Here's how the part is built. I have some questions about the finished solid (model axes, mm). Face numbers are marked on the shaded views. A direction names the side the tool comes from. Give positions to 0.01 mm unless a question says otherwise; leave off trailing zeros. Order: outer loops, then holes, each group sorted by start corner. A loop starts at its lowest first (then second) coordinate and runs counter-clockwise, first axis right, second up. Notation, with made-up numbers: (-4, 40) - (9, 40) arc R25 ccw to (9, 70) - close; hole circle Ø10 at (34.25, -3). An arc over 180 degrees is marked (long way). One line per question, with ' | ' between items.
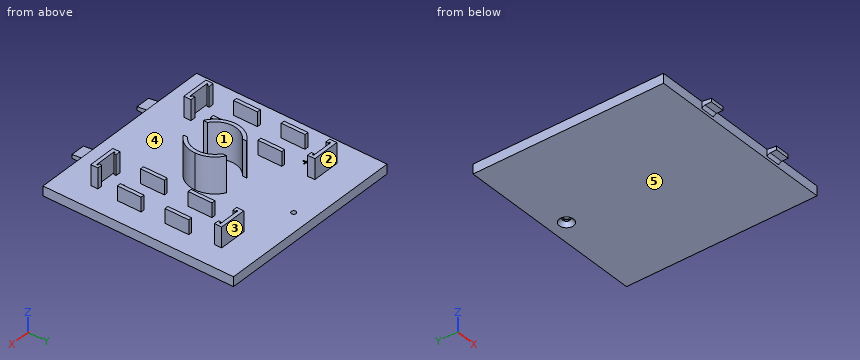
from build123d import *

# Parameters (mm, degrees)
F1_DEPTH       = 4
F2_W           = 1.5
F2_H           = 10
F3_DEPTH       = 6
F2_W_2         = 7.5
F2_H_2         = 1.5
F4_DEPTH       = 8.5
F5_R           = 1
F6_DEPTH       = 25
F7_START       = -2
F5_R_2         = 1.5
F7_DEPTH       = 23
F8_SIZE        = 1.5
F10_DEPTH      = 40
F10_DEPTH_BACK = 40
F0_W           = 20
F0_H           = 4
F0_W_2         = 28
F11_DEPTH      = 18.6
F12_DEPTH      = 0.3
F14_DEPTH      = 15


with BuildPart() as f1:
    # F0 (on Top) → F1 (new body)
    with BuildSketch(Plane.XY):
        Polygon((40, 40), (-40, 40), (-40, -40), (-20, -40), (-14, -40), (14, -40), (20, -40), (40, -40), align=None)
    extrude(amount=F1_DEPTH)

    # F2 (on face) → F3 (join)
    with BuildSketch(Plane.XY.offset(4)):
        with Locations((-30.3, -11)):
            Rectangle(F2_W, F2_H)
        with Locations((-18.2, -11)):
            Rectangle(F2_W, F2_H)
        with Locations((-18.2, 9)):
            Rectangle(F2_W, F2_H)
        with Locations((-30.3, 9)):
            Rectangle(F2_W, F2_H)
        with Locations((18.2, -11)):
            Rectangle(F2_W, F2_H)
        with Locations((18.2, 9)):
            Rectangle(F2_W, F2_H)
        with Locations((30.3, 9)):
            Rectangle(F2_W, F2_H)
        with Locations((30.3, -11)):
            Rectangle(F2_W, F2_H)
    extrude(amount=F3_DEPTH)

    # F2 (on face) → F4 (join)
    with BuildSketch(Plane.XY.offset(4)):
        Polygon((-28, 27), (-30, 27), (-30, 24), (-28, 24), (-28, 25), (-28.75, 25), (-28.75, 25.5), (-28, 25.5), align=None)
        with Locations((-24.25, 26.25)):
            Rectangle(F2_W_2, F2_H_2)
        Polygon((-18.5, 27), (-20.5, 27), (-20.5, 25.5), (-19.75, 25.5), (-19.75, 25), (-20.5, 25), (-20.5, 24), (-18.5, 24), align=None)
        Polygon((-20.5, -28), (-18.5, -28), (-18.5, -25), (-20.5, -25), (-20.5, -26), (-19.75, -26), (-19.75, -26.5), (-20.5, -26.5), align=None)
        with Locations((-24.25, -27.25)):
            Rectangle(F2_W_2, F2_H_2)
        Polygon((-30, -28), (-28, -28), (-28, -26.5), (-28.75, -26.5), (-28.75, -26), (-28, -26), (-28, -25), (-30, -25), align=None)
        Polygon((20.5, 27), (18.5, 27), (18.5, 24), (20.5, 24), (20.5, 25), (19.75, 25), (19.75, 25.5), (20.5, 25.5), align=None)
        with Locations((24.25, 26.25)):
            Rectangle(F2_W_2, F2_H_2)
        Polygon((30, 27), (28, 27), (28, 25.5), (28.75, 25.5), (28.75, 25), (28, 25), (28, 24), (30, 24), align=None)
        Polygon((28, -28), (30, -28), (30, -25), (28, -25), (28, -26), (28.75, -26), (28.75, -26.5), (28, -26.5), align=None)
        with Locations((24.25, -27.25)):
            Rectangle(F2_W_2, F2_H_2)
        Polygon((18.5, -28), (20.5, -28), (20.5, -26.5), (19.75, -26.5), (19.75, -26), (20.5, -26), (20.5, -25), (18.5, -25), align=None)
    extrude(amount=F4_DEPTH)

    # F5 (on face) → F6 (cut)
    with BuildSketch(Plane.XY.offset(4)):
        with Locations((0, 33)):
            Circle(F5_R)
    extrude(amount=-F6_DEPTH, mode=Mode.SUBTRACT)

    # F5 (on face) → F7 (cut)
    with BuildSketch(Plane.XY.offset(4).offset(F7_START)):
        with Locations((0, 33)):
            Circle(F5_R_2)
        with Locations((0, 33)):
            Circle(F5_R, mode=Mode.SUBTRACT)
    extrude(amount=-F7_DEPTH, mode=Mode.SUBTRACT)

    # F8
    f8_edges = [f1.edges().sort_by_distance(p)[0] for p in [
        (-1.5, 33, 0),
    ]]
    chamfer(f8_edges, length=F8_SIZE)

    # F9 (on Right) → F10 (join, two sides)
    with BuildSketch(Plane.YZ) as f10_sk:
        Polygon((-44, 3.5), (-44, 2), (-41.3253502548, 2), (-40, 2), (-40, 4), align=None)
        with BuildLine():
            Line((-40, 2), (-41.3253502548, 2))
            add(Edge.make_bspline(
                [(-40, 1.1688865488), (-40.1044214362, 1.3442346056), (-40.4564972437, 1.788672813), (-40.9847019479, 1.899783813), (-41.3253502548, 2)],
                knots=[0, 0, 0, 0, 0.4675971857, 1, 1, 1, 1], degree=3))
            Line((-40, 1.1688865488), (-40, 2))
        make_face()
    extrude(amount=F10_DEPTH)
    extrude(f10_sk.sketch, amount=-F10_DEPTH_BACK)

    # F0 (on Top) → F11 (cut)
    with BuildSketch(Plane.XY):
        with Locations((-30, -42)):
            Rectangle(F0_W, F0_H)
        with Locations((0, -42)):
            Rectangle(F0_W_2, F0_H)
        with Locations((30, -42)):
            Rectangle(F0_W, F0_H)
    extrude(amount=F11_DEPTH, mode=Mode.SUBTRACT)

    # F2 (on face) → F12 (cut)
    with BuildSketch(Plane.XY.offset(4)):
        Polygon((-24, 20), (-24.5, 20), (-24.5, 19), (-25.5, 19), (-25.5, 18.5), (-24.5, 18.5), (-24.5, 17.5), (-24, 17.5), (-24, 18.5), (-23, 18.5), (-23, 19), (-24, 19), align=None)
        Polygon((24.5, -18.5), (24, -18.5), (24, -19.5), (23, -19.5), (23, -20), (24, -20), (24, -21), (24.5, -21), (24.5, -20), (25.5, -20), (25.5, -19.5), (24.5, -19.5), align=None)
    extrude(amount=-F12_DEPTH, mode=Mode.SUBTRACT)

    # F13 (on face) → F14 (join)
    with BuildSketch(Plane.XY.offset(4)):
        with BuildLine():
            ThreePointArc((-5.1981253765, -7.347073742), (-9, 0), (-5.1981253765, 7.347073742))
            Line((-5.1981253765, 7.347073742), (-5.1981253765, 9.123019926))
            ThreePointArc((-5.1981253765, 9.123019926), (-10.5, 0), (-5.1981253765, -9.123019926))
            Line((-5.1981253765, -9.123019926), (-5.1981253765, -7.347073742))
        make_face()
        with BuildLine():
            ThreePointArc((5.1981253765, 7.347073742), (7.993219889, 4.136234496), (9, 0))
            ThreePointArc((9, 0), (7.993219889, -4.136234496), (5.1981253765, -7.347073742))
            Line((5.1981253765, -7.347073742), (5.1981253765, -9.123019926))
            ThreePointArc((5.1981253765, -9.123019926), (9.078279475, -5.2758735555), (10.5, 0))
            ThreePointArc((10.5, 0), (9.078279475, 5.2758735555), (5.1981253765, 9.123019926))
            Line((5.1981253765, 9.123019926), (5.1981253765, 7.347073742))
        make_face()
    extrude(amount=F14_DEPTH)


solid = f1.part
1) Thinking about a two-plate mould opening in Y: for the marked faces 3, 4 and 5, which applies, +Y half, -Y half, draft (parallel to the pull), parting line (faces both ways), or undercut?
Model answer:
face 3: +Y half | face 4: undercut | face 5: draft
2) On a 3-axis mill with a long thin cutter (end or side, diameter ignored), from which of +Z, -Z, +X, -X, +Y, -Y can I reach the whole of each face in a straight line? I mean the marked faces 1 and 2. Say none if no direction works.
Model answer:
face 1: +Z | face 2: +Z, +X, -X, +Y
3) I want a section at A-A (y = 33). List the corners of the cut face in (x, z) for me, plus the area to 3 significant figures.
Model answer:
outline: (-40, 0) - (-3, 0) - (-1.5, 1.5) - (-1.5, 2) - (-1, 2) - (-1, 4) - (-40, 4) - close; (1, 2) - (1.5, 2) - (1.5, 1.5) - (3, 0) - (40, 0) - (40, 4) - (1, 4) - close | area: 308 mm2
4) I want a section at D-D (z = 8.75). State how many separate pieces and enclosed holes the cut face has, plus the area to 3 significant figures.
Model answer:
separate pieces: 14 | enclosed holes: 0 | area: 269 mm2
5) I'm going to push flat-ended pins straight in: P1, Ø1, axis at y = 9.5, z = 6, coming from the +X side; P2, Ø5, axis at y = -14, z = 14.5, coming from the -X side; P3, Ø2.5, axis at x = 25.5, z = 6, coming from the +Y side; P4, Ø8, axis at x = -28, z = 6.5, coming from the -Y side. Where does each tip first touch, or does it pass through?
Model answer:
P1: stops at x = 31.05 | P2: passes through | P3: stops at y = 27 | P4: stops at y = -40
6) Please list where these lines run through material, in increasing order: L1, parallel to Y at x = 0, z = 1.65; L2, parallel to Y at x = 0, z = 2.9; L3, parallel to Z at x = -34, y = 26.
Model answer:
L1: y = -40 to 31.5, 34.5 to 40 | L2: y = -40 to 32, 34 to 40 | L3: z = 0 to 4
7) I want a section at B-B (z = 15.75). List the corners of the cut face in (x, y) for me, plus the area to 3 significant figures.
Model answer:
outline: (-5.2, -9.12) - (-5.2, -7.35) arc R9 cw to (-5.2, 7.35) - (-5.2, 9.12) arc R10.5 ccw to start; (5.2, -9.12) arc R10.5 ccw to (5.2, 9.12) - (5.2, 7.35) arc R9 cw to (5.2, -7.35) - close | area: 59.0 mm2
8) I want a section at C-C (x = 0). List the corners of the cut face in (y, z) for me, plus the area to 3 significant figures.
Model answer:
outline: (-40, 0) - (30, 0) - (31.5, 1.5) - (31.5, 2) - (32, 2) - (32, 4) - (-40, 4) - close; (34, 2) - (34.5, 2) - (34.5, 1.5) - (36, 0) - (40, 0) - (40, 4) - (34, 4) - close | area: 308 mm2
